Verification items for the finished model (mm, model axes). Round coordinates to 2 decimals unless told otherwise and drop trailing zeros. Loops run counter-clockwise (first coordinate to the right, second up) from the corner with the lowest first, then second, coordinate; pieces in that order, holes last. Notation, with made-up numbers: M 27.25,60 L 61.25,60 A7 cw 61.25,68 Z; hole C 18,9.25 d10. An arc over 180 degrees is marked long. Answer as CSV lines item,"result".
```python
from build123d import *

# Parameters (mm, degrees)
F0_R     = 2.54
F1_DEPTH = 5.08
F3_DEPTH = 5.08


with BuildPart() as f1:
    # F0 (on Front) → F1 (new body)
    with BuildSketch(Plane.XZ):
        with BuildLine():
            ThreePointArc((-30.166206, -46.664449), (-23.31305, -47.812995), (-19.511088, -41.996638))
            ThreePointArc((-19.511088, -41.996638), (-20.044732, -39.4486), (-21.55597, -37.328828))
            ThreePointArc((-21.55597, -37.328828), (-30.528899, -37.69152), (-30.166206, -46.664449))
        make_face()
        with Locations((-25.861088, -41.996638)):
            Circle(F0_R, mode=Mode.SUBTRACT)
        with BuildLine():
            ThreePointArc((-30.166206, -46.664449), (-30.528899, -37.69152), (-21.55597, -37.328828))
            Line((-21.55597, -37.328828), (-86.90532, 22.942827))
            ThreePointArc((-86.90532, 22.942827), (-85.394082, 20.823055), (-84.860439, 18.275017))
            ThreePointArc((-84.860439, 18.275017), (-88.6624, 12.45866), (-95.515557, 13.607206))
            Line((-95.515557, 13.607206), (-30.166206, -46.664449))
        make_face()
        with BuildLine():
            ThreePointArc((-84.860439, 18.275017), (-85.394082, 20.823055), (-86.90532, 22.942827))
            ThreePointArc((-86.90532, 22.942827), (-95.878249, 22.580135), (-95.515557, 13.607206))
            ThreePointArc((-95.515557, 13.607206), (-88.6624, 12.45866), (-84.860439, 18.275017))
        make_face()
        with Locations((-91.210439, 18.275017)):
            Circle(F0_R, mode=Mode.SUBTRACT)
    extrude(amount=F1_DEPTH)

    # F2 (on face) → F3 (join)
    with BuildSketch(Plane.XZ.offset(5.08)):
        with BuildLine():
            ThreePointArc((-95.515557, 13.607206), (-95.878249, 22.580135), (-86.90532, 22.942827))
            Line((-86.90532, 22.942827), (-124.247806, 57.383773))
            Line((-124.247806, 57.383773), (-132.858043, 48.048152))
            Line((-132.858043, 48.048152), (-95.515557, 13.607206))
        make_face()
    extrude(amount=-F3_DEPTH)


solid = f1.part
```
1) Draft check along Z on faces 1 (the cylindrical face through (-27.733, -2.504, -40.28)), 2 (the flat face through (-128.493, -2.576, 52.781)), 3 (the flat face through (-76, 0, 5)), 4 (the cylindrical face through (-88.864, -2.504, 17.302)). Enter one of: +Z half, -Z half, draft (parallel to the pull), parting line (faces both ways), or undercut.
Here are the results:
face 1,"undercut"
face 2,"+Z half"
face 3,"draft"
face 4,"undercut"
2) Section check A-A (z = 17). Record the cut outline in (x, y).
Here are the results:
outline,"M -99.19,-5.08 L -93.41,-5.08 L -93.41,0 L -99.19,0 Z; M -89.01,-5.08 L -80.46,-5.08 L -80.46,0 L -89.01,0 Z"
3) Section check B-B (x = -92). Record the cut outline in (y, z).
Here are the results:
outline,"M -5.08,10.36 L 0,10.36 L 0,15.86 L -5.08,15.86 Z; M -5.08,20.69 L 0,20.69 L 0,27.64 L -5.08,27.64 Z"
4) Go/stop test with flat-tipped pins: pin 1 (8 mm diameter, centred on x = -91.21, z = 18.28, fed in from -Y); pin 2 (1.5 mm diameter, centred on x = -68.5, y = -2, fed in from +Z); pin 3 (4 mm diameter, centred on x = -109, z = 22, fed in from +Y). Record where each tip stops, or that it passes through.
Here are the results:
pin 1,"stops at y = -5.08"
pin 2,"stops at z = 6.66"
pin 3,"passes through"
5) Section check D-D (x = -41.5). Record the cut outline in (y, z), plus the area to 3 significant figures.
Here are the results:
outline,"M -5.08,-36.21 L 0,-36.21 L 0,-18.93 L -5.08,-18.93 Z"
area,"87.8 mm^2"
6) Material ranges on probe 1 along Z at (x, y) = (-53, -2.1); probe 2 along Z at (x, y) = (-80, -3.15); probe 3 along X at (y, z) = (-0.35, -12), recorded low to high.
Here are the results:
probe 1,"z = -25.6 to -8.33"
probe 2,"z = -0.7 to 16.57"
probe 3,"x = -67.75 to -49.02"
7) Section check C-C (y = -2.3). Record the cut outline in (x, z), plus the area to 3 significant figures.
Here are the results:
outline,"M -132.86,48.05 L -30.17,-46.66 A6.35 ccw -21.56,-37.33 L -124.25,57.38 Z; hole C -91.21,18.28 d5.08; hole C -25.86,-42 d5.08"
area,"1,800 mm^2"
